Could you check a few things on this model? Use its own coordinates, in mm. A direction names the side the tool comes from. Round coordinates to 2 decimals unless told otherwise and drop trailing zeros. Loops run counter-clockwise (first coordinate to the right, second up) from the corner with the lowest first, then second, coordinate; pieces in that order, holes last.
from build123d import *

# Parameters (mm, degrees)
BOSS_EXTRUDE2_DEPTH   = 18
BOSS_EXTRUDE2_2_DEPTH = 18
BOSS_EXTRUDE2_3_DEPTH = 18
BOSS_EXTRUDE2_4_DEPTH = 18
BOSS_EXTRUDE2_5_DEPTH = 18
BOSS_EXTRUDE2_6_DEPTH = 18
BOSS_EXTRUDE3_DEPTH   = 9
SKETCH2_R             = 7
SKETCH2_R_2           = 4.5
CUT_EXTRUDE1_DEPTH    = 9
SKETCH2_3_R           = 4.5
CUT_EXTRUDE2_DEPTH    = 18
CUT_EXTRUDE3_START    = -9
CUT_EXTRUDE3_DEPTH    = 9


with BuildPart() as part:
    # Sketch1 → Boss-Extrude2 (new body)
    with BuildSketch(Plane(origin=(0, 0, 0), x_dir=(1, 0, 0), z_dir=(0, 1, 0))):
        with BuildLine():
            ThreePointArc((-6.227118887, 26.785686296), (0, 27.5), (6.227118887, 26.785686296))
            Line((6.227118887, 26.785686296), (25.649824452, 60.426799156))
            Line((25.649824452, 60.426799156), (25.956463368, 63.931698002))
            ThreePointArc((25.956463368, 63.931698002), (0, 69), (-25.956463368, 63.931698002))
            Line((-25.956463368, 63.931698002), (-25.649824452, 60.426799156))
            Line((-25.649824452, 60.426799156), (-6.227118887, 26.785686296))
        make_face()
    extrude(amount=BOSS_EXTRUDE2_DEPTH)



with BuildPart() as body_2:
    # Sketch1 → Boss-Extrude2 2 (new body)
    with BuildSketch(Plane(origin=(0, 0, 0), x_dir=(1, 0, 0), z_dir=(0, 1, 0))):
        with BuildLine():
            Line((26.310644234, 8), (65.156055364, 8))
            Line((65.156055364, 8), (68.344706261, 9.486892332))
            ThreePointArc((68.344706261, 9.486892332), (59.755752861, 34.5), (42.388242893, 54.44480567))
            Line((42.388242893, 54.44480567), (39.506230912, 52.426799156))
            Line((39.506230912, 52.426799156), (20.083525347, 18.785686296))
            ThreePointArc((20.083525347, 18.785686296), (23.815698604, 13.75), (26.310644234, 8))
        make_face()
    extrude(amount=BOSS_EXTRUDE2_2_DEPTH)


with BuildPart() as body_3:
    # Sketch1 → Boss-Extrude2 3 (new body)
    with BuildSketch(Plane(origin=(0, 0, 0), x_dir=(1, 0, 0), z_dir=(0, 1, 0))):
        with BuildLine():
            ThreePointArc((26.310644234, -8), (23.815698604, -13.75), (20.083525347, -18.785686296))
            Line((20.083525347, -18.785686296), (39.506230912, -52.426799156))
            Line((39.506230912, -52.426799156), (42.388242893, -54.44480567))
            ThreePointArc((42.388242893, -54.44480567), (59.755752861, -34.5), (68.344706261, -9.486892332))
            Line((68.344706261, -9.486892332), (65.156055364, -8))
            Line((65.156055364, -8), (26.310644234, -8))
        make_face()
    extrude(amount=BOSS_EXTRUDE2_3_DEPTH)


with BuildPart() as body_4:
    # Sketch1 → Boss-Extrude2 4 (new body)
    with BuildSketch(Plane(origin=(0, 0, 0), x_dir=(1, 0, 0), z_dir=(0, 1, 0))):
        with BuildLine():
            Line((25.649824452, -60.426799156), (6.227118887, -26.785686296))
            ThreePointArc((6.227118887, -26.785686296), (0, -27.5), (-6.227118887, -26.785686296))
            Line((-6.227118887, -26.785686296), (-25.649824452, -60.426799156))
            Line((-25.649824452, -60.426799156), (-25.956463368, -63.931698002))
            ThreePointArc((-25.956463368, -63.931698002), (0, -69), (25.956463368, -63.931698002))
            Line((25.956463368, -63.931698002), (25.649824452, -60.426799156))
        make_face()
    extrude(amount=BOSS_EXTRUDE2_4_DEPTH)


with BuildPart() as body_5:
    # Sketch1 → Boss-Extrude2 5 (new body)
    with BuildSketch(Plane(origin=(0, 0, 0), x_dir=(1, 0, 0), z_dir=(0, 1, 0))):
        with BuildLine():
            Line((-39.506230912, -52.426799156), (-20.083525347, -18.785686296))
            ThreePointArc((-20.083525347, -18.785686296), (-23.815698604, -13.75), (-26.310644234, -8))
            Line((-26.310644234, -8), (-65.156055364, -8))
            Line((-65.156055364, -8), (-68.344706261, -9.486892332))
            ThreePointArc((-68.344706261, -9.486892332), (-59.755752861, -34.5), (-42.388242893, -54.44480567))
            Line((-42.388242893, -54.44480567), (-39.506230912, -52.426799156))
        make_face()
    extrude(amount=BOSS_EXTRUDE2_5_DEPTH)


with BuildPart() as body_6:
    # Sketch1 → Boss-Extrude2 6 (new body)
    with BuildSketch(Plane(origin=(0, 0, 0), x_dir=(1, 0, 0), z_dir=(0, 1, 0))):
        with BuildLine():
            Line((-65.156055364, 8), (-26.310644234, 8))
            ThreePointArc((-26.310644234, 8), (-23.815698604, 13.75), (-20.083525347, 18.785686296))
            Line((-20.083525347, 18.785686296), (-39.506230912, 52.426799156))
            Line((-39.506230912, 52.426799156), (-42.388242893, 54.44480567))
            ThreePointArc((-42.388242893, 54.44480567), (-59.755752861, 34.5), (-68.344706261, 9.486892332))
            Line((-68.344706261, 9.486892332), (-65.156055364, 8))
        make_face()
    extrude(amount=BOSS_EXTRUDE2_6_DEPTH)


with BuildPart() as part_1:
    add(part.part)

    add(body_2.part)  # Boss-Extrude3 merges body 2

    add(body_3.part)  # Boss-Extrude3 merges body 3

    add(body_4.part)  # Boss-Extrude3 merges body 4

    add(body_5.part)  # Boss-Extrude3 merges body 5

    add(body_6.part)  # Boss-Extrude3 merges body 6
    # Sketch1_3 → Boss-Extrude3 (add)
    with BuildSketch(Plane(origin=(0, 0, 0), x_dir=(1, 0, 0), z_dir=(0, 1, 0))):
        with BuildLine():
            ThreePointArc((6.227118887, 26.785686296), (13.75, 23.815698604), (20.083525347, 18.785686296))
            Line((20.083525347, 18.785686296), (39.506230912, 52.426799156))
            Line((39.506230912, 52.426799156), (25.649824452, 60.426799156))
            Line((25.649824452, 60.426799156), (6.227118887, 26.785686296))
        make_face()
        with BuildLine():
            Line((-39.506230912, 52.426799156), (-20.083525347, 18.785686296))
            ThreePointArc((-20.083525347, 18.785686296), (-13.75, 23.815698604), (-6.227118887, 26.785686296))
            Line((-6.227118887, 26.785686296), (-25.649824452, 60.426799156))
            Line((-25.649824452, 60.426799156), (-39.506230912, 52.426799156))
        make_face()
        with BuildLine():
            Line((-65.156055364, -8), (-26.310644234, -8))
            ThreePointArc((-26.310644234, -8), (-27.5, 0), (-26.310644234, 8))
            Line((-26.310644234, 8), (-65.156055364, 8))
            Line((-65.156055364, 8), (-65.156055364, -8))
        make_face()
        with BuildLine():
            Line((-25.649824452, -60.426799156), (-6.227118887, -26.785686296))
            ThreePointArc((-6.227118887, -26.785686296), (-13.75, -23.815698604), (-20.083525347, -18.785686296))
            Line((-20.083525347, -18.785686296), (-39.506230912, -52.426799156))
            Line((-39.506230912, -52.426799156), (-25.649824452, -60.426799156))
        make_face()
        with BuildLine():
            ThreePointArc((27.5, 0), (27.201035977, -4.043963623), (26.310644234, -8))
            Line((26.310644234, -8), (65.156055364, -8))
            Line((65.156055364, -8), (65.156055364, 8))
            Line((65.156055364, 8), (26.310644234, 8))
            ThreePointArc((26.310644234, 8), (27.201035977, 4.043963623), (27.5, 0))
        make_face()
        with BuildLine():
            Line((39.506230912, -52.426799156), (20.083525347, -18.785686296))
            ThreePointArc((20.083525347, -18.785686296), (13.75, -23.815698604), (6.227118887, -26.785686296))
            Line((6.227118887, -26.785686296), (25.649824452, -60.426799156))
            Line((25.649824452, -60.426799156), (39.506230912, -52.426799156))
        make_face()
    extrude(amount=BOSS_EXTRUDE3_DEPTH)

    # Sketch2 → Cut-Extrude1 (cut)
    # profile 1 of 6: a face of its own
    with BuildSketch(Plane(origin=(0, 18, 0), x_dir=(1, 0, 0), z_dir=(0, 1, 0))):
        with Locations(Location((0, 40, 0), (0, 0, 270))):
            Circle(SKETCH2_R)
        with Locations(Location((0, 40, 0), (0, 0, 270))):
            Circle(SKETCH2_R_2, mode=Mode.SUBTRACT)
    # profile 2 of 6: a face of its own
    with BuildSketch(Plane(origin=(0, 18, 0), x_dir=(1, 0, 0), z_dir=(0, 1, 0))):
        with Locations(Location((34.641016151, 20, 0), (0, 0, 270))):
            Circle(SKETCH2_R)
        with Locations(Location((34.641016151, 20, 0), (0, 0, 270))):
            Circle(SKETCH2_R_2, mode=Mode.SUBTRACT)
    # profile 3 of 6: a face of its own
    with BuildSketch(Plane(origin=(0, 18, 0), x_dir=(1, 0, 0), z_dir=(0, 1, 0))):
        with Locations(Location((34.641016151, -20, 0), (0, 0, 270))):
            Circle(SKETCH2_R)
        with Locations(Location((34.641016151, -20, 0), (0, 0, 270))):
            Circle(SKETCH2_R_2, mode=Mode.SUBTRACT)
    # profile 4 of 6: a face of its own
    with BuildSketch(Plane(origin=(0, 18, 0), x_dir=(1, 0, 0), z_dir=(0, 1, 0))):
        with Locations(Location((0, -40, 0), (0, 0, 270))):
            Circle(SKETCH2_R)
        with Locations(Location((0, -40, 0), (0, 0, 270))):
            Circle(SKETCH2_R_2, mode=Mode.SUBTRACT)
    # profile 5 of 6: a face of its own
    with BuildSketch(Plane(origin=(0, 18, 0), x_dir=(1, 0, 0), z_dir=(0, 1, 0))):
        with Locations(Location((-34.641016151, -20, 0), (0, 0, 270))):
            Circle(SKETCH2_R)
        with Locations(Location((-34.641016151, -20, 0), (0, 0, 270))):
            Circle(SKETCH2_R_2, mode=Mode.SUBTRACT)
    # profile 6 of 6: a face of its own
    with BuildSketch(Plane(origin=(0, 18, 0), x_dir=(1, 0, 0), z_dir=(0, 1, 0))):
        with Locations(Location((-34.641016151, 20, 0), (0, 0, 270))):
            Circle(SKETCH2_R)
        with Locations(Location((-34.641016151, 20, 0), (0, 0, 270))):
            Circle(SKETCH2_R_2, mode=Mode.SUBTRACT)
    extrude(amount=-CUT_EXTRUDE1_DEPTH, mode=Mode.SUBTRACT)

    # Sketch2_3 → Cut-Extrude2 (cut)
    with BuildSketch(Plane(origin=(0, 18, 0), x_dir=(1, 0, 0), z_dir=(0, 1, 0))):
        with Locations(Location((0, 40, 0), (0, 0, 270))):
            Circle(SKETCH2_3_R)
        with Locations(Location((34.641016151, 20, 0), (0, 0, 270))):
            Circle(SKETCH2_3_R)
        with Locations(Location((34.641016151, -20, 0), (0, 0, 270))):
            Circle(SKETCH2_3_R)
        with Locations(Location((0, -40, 0), (0, 0, 270))):
            Circle(SKETCH2_3_R)
        with Locations(Location((-34.641016151, -20, 0), (0, 0, 270))):
            Circle(SKETCH2_3_R)
        with Locations(Location((-34.641016151, 20, 0), (0, 0, 270))):
            Circle(SKETCH2_3_R)
    extrude(amount=-CUT_EXTRUDE2_DEPTH, mode=Mode.SUBTRACT)

    # Sketch6 → Cut-Extrude3 (cut)
    with BuildSketch(Plane(origin=(0, 18, 0), x_dir=(1, 0, 0), z_dir=(0, 1, 0)).offset(CUT_EXTRUDE3_START)):
        with BuildLine():
            Line((-2.904975886, 55.430241959), (-3.244829287, 61.915031155))
            Line((-3.244829287, 61.915031155), (10.769094499, 68.154432018))
            ThreePointArc((10.769094499, 68.154432018), (-6.426065226, 68.700114161), (-23.221743582, 64.975))
            ThreePointArc((-23.221743582, 64.975), (0, 51.75), (23.221743582, 64.975))
            ThreePointArc((23.221743582, 64.975), (21.519668206, 65.558400532), (19.802959741, 66.097222222))
            ThreePointArc((19.802959741, 66.097222222), (9.99157553, 57.479870277), (-2.904975886, 55.430241959))
        make_face()
        with BuildLine():
            Line((-46.551509731, -30.230903894), (-51.997575213, -33.767620171))
            Line((-51.997575213, -33.767620171), (-64.408016757, -24.750906597))
            ThreePointArc((-64.408016757, -24.750906597), (-56.283011493, -39.915192813), (-44.65912882, -52.598119862))
            ThreePointArc((-44.65912882, -52.598119862), (-44.816814646, -25.875), (-67.880872402, -12.376880138))
            ThreePointArc((-67.880872402, -12.376880138), (-67.535074395, -14.142620919), (-67.143353435, -15.898744905))
            ThreePointArc((-67.143353435, -15.898744905), (-54.774815631, -20.086976906), (-46.551509731, -30.230903894))
        make_face()
        with BuildLine():
            Line((49.456485617, -25.199338065), (55.2424045, -28.147410984))
            Line((55.2424045, -28.147410984), (53.638922259, -43.40352542))
            ThreePointArc((53.638922259, -43.40352542), (62.709076719, -28.784921348), (67.880872402, -12.376880138))
            ThreePointArc((67.880872402, -12.376880138), (44.816814646, -25.875), (44.65912882, -52.598119862))
            ThreePointArc((44.65912882, -52.598119862), (46.015406189, -51.415779613), (47.340393693, -50.198477317))
            ThreePointArc((47.340393693, -50.198477317), (44.783240101, -37.392893372), (49.456485617, -25.199338065))
        make_face()
    extrude(amount=CUT_EXTRUDE3_DEPTH, mode=Mode.SUBTRACT)


solid = part_1.part
Item 1: If I drill on line 1 along X through (y, z) = (10, -47.5); line 2 along X through (y, z) = (2.25, -20); line 3 along X through (y, z) = (13.5, 25.5), over which ranges is the centre line in solid material (lowest first)?
Results list:
line 1: x = -50.05 to -36.66, -18.19 to 18.19, 36.66 to 50.05
line 2: x = -66.04 to -39.14, -30.14 to -18.87, 18.87 to 30.14, 39.14 to 66.04
line 3: x = -63.38 to -49.23, -45.04 to -38.97, -30.31 to -23.96, 23.96 to 30.31, 38.97 to 45.04, 49.23 to 50.05
Item 2: If we section it at B-B, the plane z = -4.5: Please give me the cut outline in (x, y).
Results list:
outline: (-65.16, 0) - (-27.13, 0) - (-27.13, 9) - (-65.16, 9) - close; (27.13, 0) - (65.16, 0) - (65.16, 9) - (27.13, 9) - close
Item 3: Will these pins go through, and if not, where does the flat tip stop? pin 1 (22.5 mm diameter, centred on x = 34.64, z = 20, fed in from +Y); pin 2 (13 mm diameter, centred on x = -45, z = 0.5, fed in from +Y); pin 3 (7 mm diameter, centred on x = -48, y = 15.5, fed in from -Z); pin 4 (3 mm diameter, centred on x = -38, y = 2.5, fed in from -Z).
Results list:
pin 1: stops at y = 18
pin 2: stops at y = 9
pin 3: stops at z = -52.73
pin 4: stops at z = -54.16
Item 4: We'd pull the mould along Z, two halves only. Please class faces 4 (the flat face through (-46, 9, 0)), 5 (the flat face through (0, 18, 52)): released by +Z, released by -Z, zero draft, split by the parting line, or undercut.
Results list:
face 4: undercut
face 5: zero draft
Item 5: For faces 1 (the flat face through (-23, 9, -40)), 2 (the flat face through (25.805, 8.874, 62.204)), 3 (the flat face through (46, 13, 8)), which set-ups out of +Z, -Z, +X, -X, +Y, -Y let a thin tool reach every point of the face, with its end or its side?
Results list:
face 1: +Y
face 2: +X, +Y, -Y
face 3: +X, -X, +Y
Item 6: If we section it at D-D, the plane z = 57: Please give me the cut outline in (x, y).
Results list:
outline: (-31.59, 0) - (31.59, 0) - (31.59, 9) - (23.67, 9) - (23.67, 18) - (-23.67, 18) - (-23.67, 9) - (-31.59, 9) - close
Item 7: If we section it at A-A, the plane x = 0: Count the separate pieces of the cut face and the enclosed holes in it, then the cut area to 3 significant figures.
Results list:
separate pieces: 4
enclosed holes: 0
area: 998 mm2
